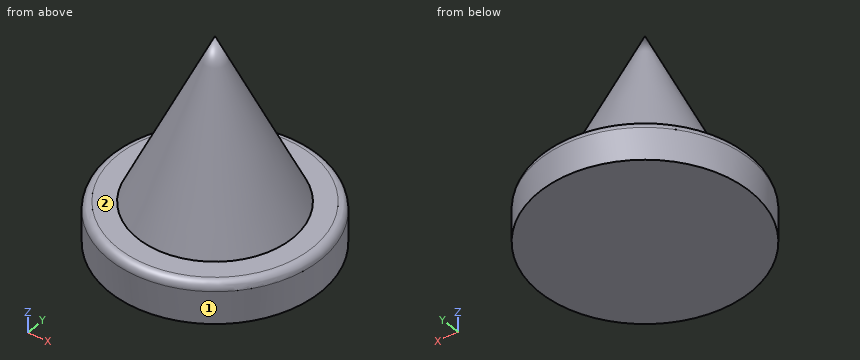
```python
from build123d import *

# Parameters (mm, degrees)
F0_R      = 65.9669270207
F1_DEPTH  = 25.4
F2_R      = 57.1573615092
F3_DEPTH  = 17.78
F4_R      = 65.9669270207
F4_R_2    = 55.5551469753
F6_DEPTH  = 65.8464431763
F7_R      = 5.08
F10_R     = 60.2787250823
F11_DEPTH = 203.2
F11_TAPER = 25


with BuildPart() as f1:
    # F0 (on Top) → F1 (new body)
    with BuildSketch(Plane.XY):
        Circle(F0_R)
    extrude(amount=F1_DEPTH)

    # F2 (on Top) → F3 (cut)
    with BuildSketch(Plane.XY):
        Circle(F2_R)
    extrude(amount=-F3_DEPTH, mode=Mode.SUBTRACT)

    # F4 (on face) → F6 (cut)
    with BuildSketch(Plane.XY.offset(25.4)):
        Circle(F4_R)
        Circle(F4_R_2, mode=Mode.SUBTRACT)
        Circle(F4_R_2)
    extrude(amount=F6_DEPTH, mode=Mode.SUBTRACT)

    # F7
    f7_edges = [f1.edges().sort_by_distance(p)[0] for p in [
        (-65.966927, 0, 25.4),
    ]]
    fillet(f7_edges, radius=F7_R)

    # F10 (on face) → F11 (join)
    with BuildSketch(Plane.XY):
        Circle(F10_R)
    extrude(amount=F11_DEPTH, taper=F11_TAPER)


solid = f1.part
```
For this review, take the finished solid that the model builds, in its own axes (mm). Face numbers are marked on the shaded views. A direction names the side the tool comes from. Round coordinates to 2 decimals unless told otherwise and drop trailing zeros. Write each loop counter-clockwise with the first axis right and the second up, starting at its lowest first coordinate (ties: lowest second). Pieces come first, ordered by that corner, then holes. Notation, with made-up numbers: (14, 48) -> (53, 48) arc R26 ccw to (53, 65) -> close; hole circle Ø10 at (6, 54). An arc over 180 degrees is marked (long way). One line per question, with ' | ' between items. Start each with the question number.
(1) Add section A-A, the plane z = 8. Write out the cut boundary in (x, y).
(2) Tool access review of the marked faces 1 and 2: name each direction out of +Z, -Z, +X, -X, +Y, -Y from which nothing blocks a thin tool from reaching the whole face with its end or side.
(3) Insertion check: P1, Ø8, axis at y = -51.5, z = 18, coming from the +X side; P2, Ø4, axis at x = -21, y = -51, coming from the +Z side; P3, Ø8, axis at x = -7.5, z = 13, coming from the +Y side. Each pin has a flat end and moves straight along its axis. Give the tip position at first contact, or say it passes through.
(4) Add section B-B, the plane z = 108. Write out the cut boundary in (x, y) (1 decimal).
(5) For line 1 along Z through (x, y) = (-30.5, -47); line 2 along X through (y, z) = (-6.5, 76.5); line 3 along X through (y, z) = (-30, 7), list the stretches that pass through material, from the lowest coordinate up. Write a range as from..to.
Answer list:
1) outline: circle Ø131.93 at (0, 0)
2) face 1: +Z, -Z | face 2: +Z
3) P1: x = 45.78 | P2: z = 25.4 | P3: y = 65.87
4) outline: circle Ø19.8 at (0, 0)
5) line 1: 0..25.4 | line 2: -23.73..23.73 | line 3: -58.75..58.75
